Check sheet for the drawn part. Datum: minimum x, y, z corner. Units: mm. A direction names the side the tool comes from. Give positions to 0.01 mm unless a question says otherwise; leave off trailing zeros. Order: outer loops, then holes, each group sorted by start corner. A loop starts at its lowest first (then second) coordinate and runs counter-clockwise, first axis right, second up. Notation, with made-up numbers: (59, 82) -> (78, 82) arc R24 ccw to (78, 105) -> close; hole circle Ø7 at (13.25, 56.25). An arc over 180 degrees is marked (long way). One line per question, with ' | ' between items. Start each with the question number.
Q1. Section check B-B on x = 31.5. Record the cut outline in (y, z).
Q2. Material ranges on probe 1 along Y at (x, z) = (26, 16.5); probe 2 along Y at (x, z) = (26, 15); probe 3 along Y at (x, z) = (8, 13.5), recorded low to high. Write a range as [from, to].
Q3. Go/stop test with a flat-tipped pin: pin 1 (3 mm diameter, centred on x = 5, z = 28, fed in from -Y). Record where the tip stops, or that it passes through.
Q4. Section check C-C on y = 18. Record the cut outline in (x, z).
Q5. Section check D-D on x = 16.5. Record the cut outline in (y, z).
Q6. Mould release check, pull along X, two halves, no side actions. Record for the marked faces 3, 4 and 5: released by +X, released by -X, zero draft, split by the parting line, or undercut.
Q7. Section check A-A on z = 16.5. Record the cut outline in (x, y), plus the area to 3 significant figures.
Q8. Access from +Z, -Z, +X, -X, +Y, -Y to the whole of each face (thin tool, end or side, straight path). Record for the marked faces 1 and 2.
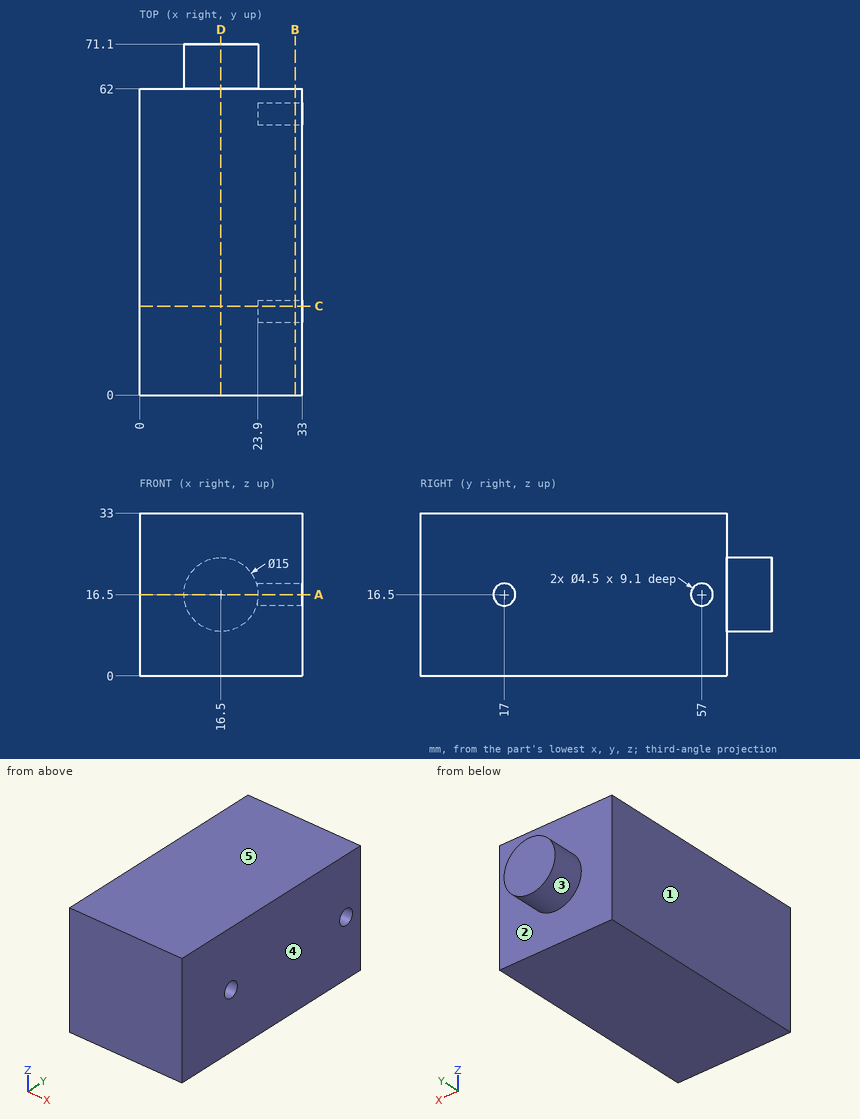
Filled in:
1) outline: (0, 0) -> (62, 0) -> (62, 33) -> (0, 33) -> close; hole circle Ø4.5 at (17, 16.5); hole circle Ø4.5 at (57, 16.5)
2) probe 1: [0, 14.75], [19.25, 54.75], [59.25, 62] | probe 2: [0, 15.32], [18.68, 55.32], [58.68, 62] | probe 3: [0, 62]
3) pin 1: y = 0
4) outline: (0, 0) -> (33, 0) -> (33, 14.48) -> (23.9, 14.48) -> (23.9, 18.52) -> (33, 18.52) -> (33, 33) -> (0, 33) -> close
5) outline: (0, 0) -> (62, 0) -> (62, 9) -> (71.1, 9) -> (71.1, 24) -> (62, 24) -> (62, 33) -> (0, 33) -> close
6) face 3: split by the parting line | face 4: released by +X | face 5: zero draft
7) outline: (0, 0) -> (33, 0) -> (33, 14.75) -> (23.9, 14.75) -> (23.9, 19.25) -> (33, 19.25) -> (33, 54.75) -> (23.9, 54.75) -> (23.9, 59.25) -> (33, 59.25) -> (33, 62) -> (24, 62) -> (24, 71.1) -> (9, 71.1) -> (9, 62) -> (0, 62) -> close | area: 2,100 mm²
8) face 1: +Z, -Z, -X, +Y, -Y | face 2: +Y
